Autodesk Inventor part; units mm, degrees
ref_plane "YZ Plane" through (0, 0, 0) normal (1, 0, 0) x (0, 1, 0)
ref_plane "XZ Plane" through (0, 0, 0) normal (0, 1, 0) x (-1, 0, 0)
ref_plane "XY Plane" through (0, 0, 0) normal (0, 0, 1) x (1, 0, 0)
sketch "Эскиз1" plane through (0, 0, 0) normal (0, 0, 1) x (1, 0, 0)
  line L0 (-42, 24) -> (-42, 23)
  line L1 (-10, 34) -> (-32, 34)
  line L2 (-42, 23) -> (-42, 0)
  line L3 (0, 23) -> (-42, 23)
  line L4 (-42, 0) -> (0, 0)
  line L5 (-42, 23) -> (0, 23)
  line L6 (-27.8, 26.9412) -> (-30.5, 25.3823)
  line L7 (-30.5, 25.3823) -> (-33.2, 26.9412)
  circle A0 centre (-30.5, 28.5) radius 1.5
  line L8 (-27.8, 30.0588) -> (-27.8, 26.9412)
  line L9 (-33.2, 26.9412) -> (-33.2, 30.0588)
  arc A1 (-32, 34) -> (-42, 24) centre (-32, 24) ccw
  line L10 (-30.5, 31.6177) -> (-27.8, 30.0588)
  line L11 (-33.2, 30.0588) -> (-30.5, 31.6177)
  line L12 (-14.2, 26.9412) -> (-14.2, 30.0588)
  line L13 (-14.2, 30.0588) -> (-11.5, 31.6177)
  line L14 (-11.5, 25.3823) -> (-14.2, 26.9412)
  circle A2 centre (-11.5, 28.5) radius 1.5
  line L15 (-11.5, 31.6177) -> (-8.8, 30.0588)
  line L16 (-8.8, 30.0588) -> (-8.8, 26.9412)
  line L17 (-8.8, 26.9412) -> (-11.5, 25.3823)
  line L18 (0, 0) -> (0, 23)
  line L19 (0, 23) -> (0, 24)
  arc A3 (0, 24) -> (-10, 34) centre (-10, 24) ccw
  dimension "d0" = 23
  dimension "d1" = 5.4
  dimension "d2" = 10
  dimension "d4" = 4
  dimension "d5" = 4
  dimension "d7" = 4
  dimension "d8" = 10
  dimension "d9" = 10
  dimension "d10" = 42
extrude "Выдавливание1" add sketch "Эскиз1" along normal blind 21 contours L3 L18 L4 L2
sketch "Эскиз2" plane through (-42, 0, 0) normal (0, -1, 0) x (1, 0, 0)
  line L0 (0, 21) -> (42, 21)
  circle A0 centre (21, 21) radius 18.1
  point P0 (42, 0)
  point P1 (39.1, 21)
  point P2 (2.9, 21)
extrude "Выдавливание2" cut sketch "Эскиз2" against normal blind 20 contours L0 A0 picked at (19.3763, 11.111)
extrude "Выдавливание3" add sketch "Эскиз1" along normal blind 3 contours A1 L1 A3 L19 L3 L0 | L6 L7 L9 L11 L10 L8 | L12 L13 L15 L16 L17 L14
chamfer "Фаска1" distance 0.3 distance2 0.1 5 edges at (0, 12, 0) (-2.9289, 31.0711, 0) (-21, 34, 0) (-39.0711, 31.0711, 0) (-21, 0, 0) measured on face at (-18.0106, 9.0325, 0)
properties part number "Держатель динамика"
Check sheet for the modelled part. Datum: model origin and axes. Units: mm. A direction names the side the tool comes from. Give positions to 0.01 mm unless a question says otherwise; leave off trailing zeros. Order: outer loops, then holes, each group sorted by start corner. A loop starts at its lowest first (then second) coordinate and runs counter-clockwise, first axis right, second up. Notation, with made-up numbers: M 40,70.5 L 45,70.5 A22 ccw 45,109.5 Z; hole C 37.25,69.5 d9. An arc over 180 degrees is marked long. Answer as CSV lines item,"result". Start each with the question number.
Item 1: Tool access check on faces 1 (the face through (-39.15, 30.99, 1.53)), 2 (the face through (-21, 23, 12)), 3 (the face through (-21.398, 9.86, 2.904)). Record the directions out of +Z, -Z, +X, -X, +Y, -Y that give a thin tool (end or side, any length) a straight path to the whole face; none if there is none.
Item 2: Gauge pin test, flat ends, axial feed: P1, Ø4, axis at x = -16.5, y = 14, coming from the +Z side; P2, Ø1.8, axis at x = -11.5, y = 28.5, coming from the +Z side; P3, Ø5.5, axis at x = -21, z = 15, coming from the +Y side; P4, Ø5.5, axis at x = -18.5, z = 7.5, coming from the -Y side. Record the tip position at first contact, or that the pin passes through.
Item 3: Cross-section at D-D on x = -11.5. Enter the section's corners in (y, z).
Item 4: Cross-section at A-A on x = -21. Enter the section's corners in (y, z), plus the area to 3 significant figures.
Item 5: Cross-section at C-C on z = 8.25. Enter the section's corners in (x, y), plus the area to 3 significant figures.
Item 6: Cross-section at B-B on y = 19.5. Enter the section's corners in (x, z).
Item 7: Thickness scan on line 1 (Y direction, x = -11.5, z = 1.2); line 2 (Z direction, x = -28.5, y = 28); line 3 (Y direction, x = -19, z = 6.5). Record the ranges inside material, lowest first. Write a range as [from, to].
Item 8: Mould release check, pull along Y, two halves, no side actions. Record for faces 4 (the face through (-3.01, 31.15, 1.53)), 5 (the face through (-11.695, 27.013, 1.479)), 6 (the face through (-31.61, 27.49, 1.48)), 7 (the face through (-42, 12, 10)): +Y half, -Y half, draft (parallel to the pull), parting line (faces both ways), or undercut.
Established:
1,face 1,"+Z, -Z, -X, +Y"
1,face 2,"+Z, +X, -X, +Y"
1,face 3,"+Z, -Y"
2,P1,"stops at z = 4.11"
2,P2,"passes through"
2,P3,"stops at y = 23"
2,P4,"stops at y = 20"
3,outline,"M 0,0.1 L 0.3,0 L 27,0 L 27,3 L 23,3 L 23,21 L 20,21 L 20,5.59 L 0,5.59 Z; M 30,0 L 33.7,0 L 34,0.1 L 34,3 L 30,3 Z"
4,outline,"M 0,0.1 L 0.3,0 L 33.7,0 L 34,0.1 L 34,3 L 23,3 L 23,21 L 20,21 L 20,2.9 L 0,2.9 Z"
4,area,"154 mm^2"
5,outline,"M -42,0 L -33.85,0 L -33.85,20 L -8.15,20 L -8.15,0 L 0,0 L 0,23 L -42,23 Z"
5,area,"452 mm^2"
6,outline,"M -42,0.1 L -41.7,0 L -0.3,0 L 0,0.1 L 0,21 L -2.9,21 A18.1 cw -39.1,21 L -42,21 Z"
7,line 1,"y = [0, 27], [30, 34]"
7,line 2,"z = [0, 3]"
7,line 3,"y = [20, 23]"
8,face 4,"+Y half"
8,face 5,"undercut"
8,face 6,"undercut"
8,face 7,"draft"
